Can you work these out from the model? Positions are in its coordinate system, mm. A direction names the side the tool comes from. Give positions to 0.01 mm unless a question says otherwise; leave off trailing zeros. Write each loop counter-clockwise with the first axis right and the second up, starting at its lowest first coordinate (ties: lowest second). Pieces come first, ordered by that corner, then holes.
```python
from build123d import *

# Parameters (mm, degrees)
F0_R     = 1.45
F1_DEPTH = 20
F3_DEPTH = 25
F5_DEPTH = 25


# Not quite as in the source:
# - a feature names something its author has since deleted; it is built from what else it names


with BuildPart() as f1:
    # F0 (on Top) → F1 (new body)
    with BuildSketch(Plane.XY):
        with BuildLine():
            Line((5.2166173299, -7.3856279958), (5.6577173299, -2.0351279958))
            Line((5.6577173299, -2.0351279958), (5.6577173299, 12.0690828189))
            ThreePointArc((5.6577173299, 12.0690828189), (5.068252548, 14.1845927754), (3.5162961604, 15.7383889255))
            ThreePointArc((3.5162961604, 15.7383889255), (2.260074285, 16.2332107279), (0.9331621041, 16.4827023722))
            ThreePointArc((0.9331621041, 16.4827023722), (2.4795483886, 15.6499153849), (3.0965173299, 14.0054720042))
            ThreePointArc((3.0965173299, 14.0054720042), (2.4482954337, 12.3259131769), (0.8397830463, 11.5173357959))
            ThreePointArc((0.8397830463, 11.5173357959), (2.7724359809, 10.8070477652), (3.6577173299, 8.9480336756))
            Line((3.6577173299, 8.9480336756), (3.6577173299, -1.9528267058))
            Line((3.6577173299, -1.9528267058), (3.2233793816, -7.2213036786))
            Line((3.2233793816, -7.2213036786), (3.0354523847, -9.5008398307))
            ThreePointArc((3.0354523847, -9.5008398307), (2.6844675314, -10.7628559885), (2.1688231186, -11.9670096287))
            ThreePointArc((2.1688231186, -11.9670096287), (2.8315798002, -16.3061539408), (6.1209868425, -13.3997435963))
            ThreePointArc((6.1209868425, -13.3997435963), (5.5965527788, -12.467225095), (5.2166173299, -11.4670896557))
            Line((5.2166173299, -11.4670896557), (5.2166173299, -7.3856279958))
        make_face()
        with Locations((3.6836173299, -13.9558279958)):
            Circle(F0_R, mode=Mode.SUBTRACT)
        with BuildLine():
            ThreePointArc((0.5965173299, 16.5054720042), (0.7649742372, 16.4960760435), (0.9331621041, 16.4827023722))
            ThreePointArc((0.9331621041, 16.4827023722), (0.7652242949, 16.4997731007), (0.5965173299, 16.5054720042))
        make_face()
        with BuildLine():
            ThreePointArc((3.0965173299, 14.0054720042), (2.4795483886, 15.6499153849), (0.9331621041, 16.4827023722))
            ThreePointArc((0.9331621041, 16.4827023722), (0.7649742372, 16.4960760435), (0.5965173299, 16.5054720042))
            ThreePointArc((0.5965173299, 16.5054720042), (-1.903159389, 13.9652687601), (0.6769134206, 11.5067650449))
            ThreePointArc((0.6769134206, 11.5067650449), (0.7582691412, 11.5132690403), (0.8397830463, 11.5173357959))
            ThreePointArc((0.8397830463, 11.5173357959), (2.4482954337, 12.3259131769), (3.0965173299, 14.0054720042))
        make_face()
        with Locations((0.5965173299, 14.0054720042)):
            Circle(F0_R, mode=Mode.SUBTRACT)
        with BuildLine():
            ThreePointArc((0.6769134206, 11.5067650449), (0.7584345203, 11.5107209498), (0.8397830463, 11.5173357959))
            ThreePointArc((0.8397830463, 11.5173357959), (0.7582691412, 11.5132690403), (0.6769134206, 11.5067650449))
        make_face()
    extrude(amount=F1_DEPTH)

    # F2 (on face) → F3 (cut)
    with BuildSketch(Plane.YZ.offset(5.6577173299)):
        with BuildLine():
            Line((3.4114552828, 13), (3.4114552828, 15.5))
            ThreePointArc((3.4114552828, 15.5), (1.5169774116, 17.3944778712), (-0.3775004597, 15.5))
            Line((-0.3775004597, 15.5), (-0.3775004597, 13))
            ThreePointArc((-0.3775004597, 13), (1.5169774116, 11.1055221288), (3.4114552828, 13))
        make_face()
        with BuildLine():
            Line((6.6224995403, 7), (6.6224995403, 4.5))
            ThreePointArc((6.6224995403, 4.5), (8.5169774116, 2.6055221288), (10.4114552828, 4.5))
            Line((10.4114552828, 4.5), (10.4114552828, 7))
            ThreePointArc((10.4114552828, 7), (8.5169774116, 8.8944778712), (6.6224995403, 7))
        make_face()
        with BuildLine():
            ThreePointArc((10.4114552828, 15.5), (8.5169774116, 17.3944778712), (6.6224995403, 15.5))
            Line((6.6224995403, 15.5), (6.6224995403, 13))
            ThreePointArc((6.6224995403, 13), (8.5169774116, 11.1055221288), (10.4114552828, 13))
            Line((10.4114552828, 13), (10.4114552828, 15.5))
        make_face()
        with BuildLine():
            ThreePointArc((-0.3775004597, 4.5), (1.5169774116, 2.6055221288), (3.4114552828, 4.5))
            Line((3.4114552828, 4.5), (3.4114552828, 7))
            ThreePointArc((3.4114552828, 7), (1.5169774116, 8.8944778712), (-0.3775004597, 7))
            Line((-0.3775004597, 7), (-0.3775004597, 4.5))
        make_face()
    extrude(amount=-F3_DEPTH, mode=Mode.SUBTRACT)

    # F4 (on face) → F5 (cut)
    with BuildSketch(Plane(origin=(5.7861693945, -0.4770169741, 0), x_dir=(0.0821621586, 0.9966189742, 0), z_dir=(0.9966189742, -0.0821621586, 0))):
        with BuildLine():
            ThreePointArc((-2.3532448105, 15.5), (-4.2477226817, 17.3944778712), (-6.142200553, 15.5))
            Line((-6.142200553, 15.5), (-6.142200553, 13))
            ThreePointArc((-6.142200553, 13), (-4.2477226817, 11.1055221288), (-2.3532448105, 13))
            Line((-2.3532448105, 13), (-2.3532448105, 15.5))
        make_face()
        with BuildLine():
            ThreePointArc((-6.142200553, 4.5), (-4.2477226817, 2.6055221288), (-2.3532448105, 4.5))
            Line((-2.3532448105, 4.5), (-2.3532448105, 7))
            ThreePointArc((-2.3532448105, 7), (-4.2477226817, 8.8944778712), (-6.142200553, 7))
            Line((-6.142200553, 7), (-6.142200553, 4.5))
        make_face()
    extrude(amount=-F5_DEPTH, mode=Mode.SUBTRACT)


solid = f1.part
```
1) Suppose I cut it at A-A on z = 5.5. Write out the boundary of the cut face in (x, y).
Values follow:
outline: (0.84, 11.52) arc R2.73 cw to (3.13, 10.41) - (5.66, 10.41) - (5.66, 12.07) arc R4.33 ccw to (3.52, 15.74) arc R7.14 ccw to (0.93, 16.48) arc R2.5 ccw (long way) to start; (2.17, -11.97) arc R2.5 ccw (long way) to (6.12, -13.4) arc R7.17 cw to (5.22, -11.47) - (5.22, -7.39) - (5.28, -6.6) - (3.29, -6.43) - (3.04, -9.5) arc R9.83 cw to start; (3.6, -2.66) - (5.59, -2.82) - (5.66, -2.04) - (5.66, -0.38) - (3.66, -0.38) - (3.66, -1.95) - close; (3.66, 3.41) - (5.66, 3.41) - (5.66, 6.62) - (3.66, 6.62) - close; hole circle Ø2.9 at (0.6, 14.01); hole circle Ø2.9 at (3.68, -13.96)
2) Suppose I cut it at C-C on y = 1.5. Write out the boundary of the cut face in (x, z), plus the area to 3 significant figures.
Values follow:
outline: (3.66, 0) - (5.66, 0) - (5.66, 2.61) - (3.66, 2.61) - close; (3.66, 8.89) - (5.66, 8.89) - (5.66, 11.11) - (3.66, 11.11) - close; (3.66, 17.39) - (5.66, 17.39) - (5.66, 20) - (3.66, 20) - close
area: 14.8 mm2
3) Please list where these lines run through material, in increasing order: L1, parallel to Y at x = 2.5, z = 12.75; L2, parallel to Y at x = 0.5, z = 5; L3, parallel to X at y = 4, z = 18.5.
Values follow:
L1: y = -16.16 to -14.79, -13.12 to -11.25, 11.03 to 16.16
L2: y = 11.51 to 12.56, 15.45 to 16.5
L3: x = 3.66 to 5.66
4) For pin 1 Ø2 at (x, z) = (4.5, 14.5) entering from -Y; pin 2 Ø2 at (x, z) = (2.5, 6) entering from -Y; pin 3 Ø8 at (y, z) = (7, 5) entering from +X; pin 4 Ø2 at (x, z) = (4.5, 15) entering from +Y, each with a flat end and sliding along its axis, tell me the tip position at first contact or that it passes through.
Values follow:
pin 1: stops at y = -16.46
pin 2: stops at y = -16.45
pin 3: stops at x = 5.66
pin 4: stops at y = 15.75
5) For faces 1 (the face through (4.61, -2.74, 14.23)), 2 (the face through (4.692, 8.559, 8.894)), 3 (the face through (5.434, -4.748, 9.86)), which set-ups out of +Z, -Z, +X, -X, +Y, -Y let a thin tool reach every point of the face, with its end or its side?
Values follow:
face 1: -X
face 2: +X, -X
face 3: +Z, -Z, +X
6) Suppose I cut it at B-B on x = 4.5. State how many separate pieces and enclosed holes the cut face has, plus the area to 3 significant figures.
Values follow:
separate pieces: 2
enclosed holes: 6
area: 453 mm2
7) Suppose I cut it at D-D on z = 10. Write out the boundary of the cut face in (x, y).
Values follow:
outline: (0.84, 11.52) arc R2.73 cw to (3.66, 8.95) - (3.66, -1.95) - (3.04, -9.5) arc R9.83 cw to (2.17, -11.97) arc R2.5 ccw (long way) to (6.12, -13.4) arc R7.17 cw to (5.22, -11.47) - (5.22, -7.39) - (5.66, -2.04) - (5.66, 12.07) arc R4.33 ccw to (3.52, 15.74) arc R7.14 ccw to (0.93, 16.48) arc R2.5 ccw (long way) to start; hole circle Ø2.9 at (0.6, 14.01); hole circle Ø2.9 at (3.68, -13.96)
